Design review of the part built by this model. Coordinates are the model's own, in mm. A direction names the side the tool comes from. Round coordinates to 2 decimals unless told otherwise and drop trailing zeros. Loops run counter-clockwise (first coordinate to the right, second up) from the corner with the lowest first, then second, coordinate; pieces in that order, holes last. Notation, with made-up numbers: M -33,-35 L -4,-35 A12 cw -4,-24 Z; hole C 31.25,53 d5. An arc over 180 degrees is marked long. Use a Markdown table: item, result.
from build123d import *

# Parameters (mm, degrees)
AXLE_BASE_SKETCH_R        = 19
AXLE_DEPTH                = 98.5
GUARD_BASE_R              = 30
GUARD_DEPTH               = 5
INNER_AXLE_HOLE_BASE_R    = 10
INNER_AXLE_HOLE_DEPTH     = 104.5
BEND_ROOM_BASE_W          = 1.5
BEND_ROOM_BASE_H          = 50
BEND_ROOM_1_DEPTH         = 57
BEND_ROOM_2_COUNT         = 2
BEND_ROOM_2_ANGLE         = 90
EASY_REMOVAL_CHAMFER_SIZE = 4


with BuildPart() as part:
    # Axle base sketch → Axle (new body)
    with BuildSketch(Plane.XY):
        Circle(AXLE_BASE_SKETCH_R)
    extrude(amount=AXLE_DEPTH)

    # Guard base → Guard (add)
    with BuildSketch(Plane(origin=(0, 0, 0), x_dir=(-1, 0, 0), z_dir=(0, 0, -1))):
        Circle(GUARD_BASE_R)
    extrude(amount=GUARD_DEPTH)

    # Inner axle hole base → Inner axle hole (cut, through all)
    with BuildSketch(Plane.XY.offset(98.5)):
        Circle(INNER_AXLE_HOLE_BASE_R)
    extrude(amount=-INNER_AXLE_HOLE_DEPTH, mode=Mode.SUBTRACT)

    # Mate ring base → Mate rings (revolve)
    with BuildSketch(Plane(origin=(0, 0, 0), x_dir=(1, 0, 0), z_dir=(0, 1, 0))):
        Polygon((19, -98.5), (19.75, -97.75), (19.75, -97), (19, -96.25), align=None)
        Polygon((19, -92.75), (19.75, -92), (19.75, -91.25), (19, -90.5), align=None)
    revolve(axis=Axis((0, 0, 0), (0, 0, -1)))

    # Bend room base → Bend room 1 (cut)
    with BuildSketch(Plane.XY.offset(98.5)):
        Rectangle(BEND_ROOM_BASE_W, BEND_ROOM_BASE_H)
    bend_room_1 = extrude(amount=-BEND_ROOM_1_DEPTH, mode=Mode.SUBTRACT)

    # Bend room 2: Bend room 1 ×2 about axis
    bend_room_2_axis = Axis((0, 0, 0), (0, 0, -1))
    for i in range(1, BEND_ROOM_2_COUNT):
        add(bend_room_1.rotate(bend_room_2_axis, i * BEND_ROOM_2_ANGLE / (BEND_ROOM_2_COUNT - 1)), mode=Mode.SUBTRACT)

    # Easy removal chamfer
    easy_removal_chamfer_edges = [part.edges().sort_by_distance(p)[0] for p in [
        (30, 0, 0),
    ]]
    chamfer(easy_removal_chamfer_edges, length=EASY_REMOVAL_CHAMFER_SIZE)


solid = part.part
1. Take a section at B-B on z = 29. Give the boundary of the cut face in (x, y).
Check values:
| item | result |
|---|---|
| outline | C 0,0 d38; hole C 0,0 d20 |
2. Machinability: for faces 4 (the face through (-0.75, 14, 70)), 5 (the face through (14.11, -13.82, 97.37)), 6 (the face through (-13.66, 13.38, 90.62)), 7 (the face through (13.575, 13.294, 94.476)), 8 (the face through (-14, 0.75, 70)), which of the approach directions +Z, -Z, +X, -X, +Y, -Y give a long, thin tool a straight path to every point of the face, cutting with its end or side? Answer none if there is none.
Check values:
| item | result |
|---|---|
| face 4 | +Z, +Y, -Y |
| face 5 | +Z, +X, -Y |
| face 6 | -X, +Y |
| face 7 | +X, +Y |
| face 8 | +Z, +X, -X |
3. Wall thickness on line 1 along X through (y, z) = (0, 27); line 2 along X through (y, z) = (-4, 2.5): over which ranges is each line inside the solid? List them lowest first. Write a range as from..to.
Check values:
| item | result |
|---|---|
| line 1 | x = -19..-10, 10..19 |
| line 2 | x = -18.57..-9.17, 9.17..18.57 |
4. The part is to be moulded in two halves that separate along X. For faces 1 (the face through (29.97, 1.32, -4.49)), 2 (the face through (13.66, -13.38, 90.62)), 3 (the face through (0.75, 14, 70)), say which applies: pulls with the +X half, pulls with the -X half, needs draft (parallel to the pull), parting line crosses it, or undercut.
Check values:
| item | result |
|---|---|
| face 1 | parting line crosses it |
| face 2 | pulls with the +X half |
| face 3 | undercut |
5. Take a section at A-A on z = 88. Give the boundary of the cut face in (x, y), and give its area (3 significant figures).
Check values:
| item | result |
|---|---|
| outline | M -18.99,-0.75 A19 ccw -0.75,-18.99 L -0.75,-9.97 A10 cw -9.97,-0.75 Z; M -18.99,0.75 L -9.97,0.75 A10 cw -0.75,9.97 L -0.75,18.99 A19 ccw Z; M 0.75,-18.99 A19 ccw 18.99,-0.75 L 9.97,-0.75 A10 cw 0.75,-9.97 Z; M 0.75,9.97 A10 cw 9.97,0.75 L 18.99,0.75 A19 ccw 0.75,18.99 Z |
| area | 766 mm² |
6. Insertion check: pin 1 (1.2 mm diameter, centred on x = 0, y = 13, fed in from +Z); pin 2 (3 mm diameter, centred on x = -14, z = 68, fed in from -Y); pin 3 (8 mm diameter, centred on x = -15.5, z = 82.5, fed in from +Y); pin 4 (6 mm diameter, centred on y = 23.5, z = 12.5, fed in from +X). Each pin has a flat end and moves straight along its axis. Give the tip position at first contact, or say it passes through.
Check values:
| item | result |
|---|---|
| pin 1 | stops at z = 41.5 |
| pin 2 | stops at y = -14.31 |
| pin 3 | stops at y = 15.12 |
| pin 4 | passes through |
